The listing builds one solid part. Answer for the finished solid, in the listing's coordinates (mm). Face numbers are marked on the shaded views. A direction names the side the tool comes from. Coordinates: 2 decimals unless noted, no trailing zeros. Order: outer loops, then holes, each group sorted by start corner. A loop starts at its lowest first (then second) coordinate and runs counter-clockwise, first axis right, second up. Notation, with made-up numbers: (43.5, 17) - (100.5, 17) arc R30 cw to (100.5, 44) - close; hole circle Ø10 at (6, -7.5). An arc over 180 degrees is marked (long way). Use a Markdown table: item, result. Add a question column.
Item 1: The part is cut by section D-D, the plane y = 58. Give the vertices of the cut face in (x, z), then the cut area to 3 significant figures.
Item 2: For the marked faces 1 and 2, determine the directions among +Z, -Z, +X, -X, +Y, -Y from which every point of the face is accessible in a straight line to the end or side of a thin tool.
Item 3: Flat-ended cylindrical pins translate along their axes: P1, Ø2, axis at x = -14.5, y = -2.5, coming from the +Z side; P2, Ø3, axis at y = 53.5, z = 11.5, coming from the -X side; P3, Ø6, axis at x = -13.5, y = 6.5, coming from the +Z side. Find the tip coordinate at first contact, or state that the pin passes through.
Item 4: Find the intervals of material crossed by line 1 along Y through (x, z) = (16, -6.5); line 2 along Y through (x, z) = (22, 12); line 3 along X through (y, z) = (5, 3.5), in increasing order.
Item 5: The part is cut by section C-C, the plane y = 0. Give the vertices of the cut face in (x, z).
from build123d import *

# Parameters (mm, degrees)
F0_R     = 35
F1_DEPTH = 12.5
F2_R     = 5
F3_SIZE  = 19.99999
F4_R     = 14.7680159512
F5_DEPTH = 55


# Not quite as in the source:
# - a fillet or chamfer is up to 0.001 mm smaller than in the source, because OpenCascade refuses the exact size


with BuildPart() as f1:
    # F0 (on Front) → F1 (new body, symmetric)
    with BuildSketch(Plane.XZ):
        Circle(F0_R)
    extrude(amount=F1_DEPTH, both=True)

    # F2
    f2_edges = [f1.edges().sort_by_distance(p)[0] for p in [
        (-35, -12.5, 0),
    ]]
    fillet(f2_edges, radius=F2_R)

    # F3 (size 20 in the source; OpenCascade refuses exactly that, so slightly less here)
    f3_edges = [f1.edges().sort_by_distance(p)[0] for p in [
        (-35, 12.5, 0),
    ]]
    chamfer(f3_edges, length=F3_SIZE)

    # F4 (on face) → F5 (join)
    with BuildSketch(Plane(origin=(0, 12.5, 0), x_dir=(-1, 0, 0), z_dir=(0, 1, 0))):
        Circle(F4_R)
    extrude(amount=F5_DEPTH)


solid = f1.part
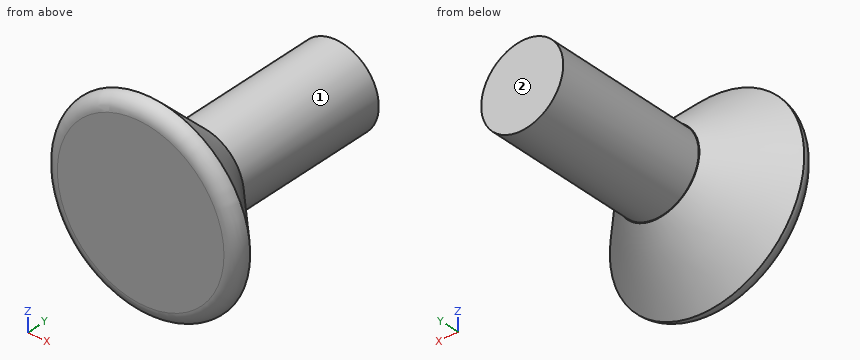
Solution:
| question | item | result |
|---|---|---|
| 1 | outline | circle Ø29.54 at (0, 0) |
| 1 | area | 685 mm2 |
| 2 | face 1 | +Y |
| 2 | face 2 | +Z, -Z, +X, -X, +Y |
| 3 | P1 | stops at z = 27.51 |
| 3 | P2 | stops at x = -10.87 |
| 3 | P3 | stops at z = 20.32 |
| 4 | line 1 | y = -12.5 to 10.23 |
| 4 | line 2 | y = -12.5 to 2.44 |
| 4 | line 3 | x = -22.23 to 22.23 |
| 5 | outline | circle Ø55 at (0, 0) |
